Check sheet for the modelled part. Datum: model origin and axes. Units: mm. A direction names the side the tool comes from. Coordinates: 2 decimals unless noted, no trailing zeros. Write each loop counter-clockwise with the first axis right and the second up, starting at its lowest first coordinate (ties: lowest second). Pieces come first, ordered by that corner, then holes. Notation, with made-up numbers: (-12.75, -36.5) -> (-7.75, -36.5) arc R15 ccw to (-7.75, -27.5) -> close; hole circle Ø3 at (38.5, 28.25). An arc over 180 degrees is marked (long way). One line per item, written item: value. Start each with the question number.
1) Sectioned sample at C-C on z = -5. Enter the section's corners in (x, y).
2) Scan lines: line 1 along X through (y, z) = (14.5, -54.5); line 2 along X through (y, z) = (18, -39); line 3 along Y through (x, z) = (21.5, -45). Record each from-to range of solid material in increasing order. Write a range as [from, to].
3) Draft check along X on faces 1 (the flat face through (24, 35, -60.5)), 2 (the cylindrical face through (18.082, 14.392, -23.825)), 3 (the cylindrical face through (7.114, 14.392, -25.069)). Enter one of: +X half, -X half, draft (parallel to the pull), parting line (faces both ways), or undercut.
4) Sectioned sample at A-A on y = 34.5. Enter the section's corners in (x, z), plus the area to 3 significant figures.
5) Gauge pin test, flat ends, axial feed: P1, Ø4, axis at x = 45.5, z = -43, coming from the +Y side; P2, Ø1.5, axis at y = 51, z = -42, coming from the +X side; P3, Ø6.5, axis at x = 49.15, y = 18.55, coming from the +Z side. Record the tip position at first contact, or that the pin passes through.
6) Set-up check for faces 4 (the flat face through (14.65, 14.39, -25.02)), 5 (the flat face through (51, 5, -47)), 6 (the flat face through (16, 24.05, -52)): record each of +Z, -Z, +X, -X, +Y, -Y from which the full face is reachable in a straight line by a thin tool's end or side.
7) Sectioned sample at B-B on x = 11.5. Enter the section's corners in (y, z), plus the area to 3 significant figures.
```python
from build123d import *

# Parameters (mm, degrees)
BOSS_EXTRUDE1_DEPTH = 5
BOSS_EXTRUDE2_DEPTH = 5
BOSS_EXTRUDE3_DEPTH = 5
SKETCH6_R           = 2.5
CUT_EXTRUDE1_DEPTH  = 107.549284371
BOSS_EXTRUDE4_DEPTH = 19.05
SKETCH9_R           = 5.5
SKETCH9_R_2         = 2.5
BOSS_EXTRUDE5_DEPTH = 25.4


with BuildPart() as part:
    # Sketch1 → Boss-Extrude1 (new body)
    with BuildSketch(Plane(origin=(0, 0, 0), x_dir=(1, 0, 0), z_dir=(0, 1, 0))):
        Polygon((0, 0), (0, 60.5), (60.5, 60.5), (60.5, 47.75), (12.75, 0), align=None)
    extrude(amount=BOSS_EXTRUDE1_DEPTH)

    # Sketch4 → Boss-Extrude2 (add)
    with BuildSketch(Plane.ZY):
        Polygon((-60.5, 5), (-60.5, 68.5), (-19.4, 68.5), (0, 10.308629506), (0, 5), align=None)
    extrude(amount=-BOSS_EXTRUDE2_DEPTH)

    # Sketch5 → Boss-Extrude3 (add)
    with BuildSketch(Plane(origin=(0, 0, -60.5), x_dir=(-1, 0, 0), z_dir=(0, 0, -1))):
        Polygon((-5, 5), (-5, 68.5), (-41, 68.5), (-60.5, 10.004653177), (-60.5, 5), align=None)
    extrude(amount=-BOSS_EXTRUDE3_DEPTH)

    # Sketch6 → Cut-Extrude1 (cut, through all)
    with BuildSketch(Plane(origin=(0, 5, 0), x_dir=(1, 0, 0), z_dir=(0, 1, 0))):
        with Locations(Location((16.5, 15, 0), (0, 0, 270))):
            Circle(SKETCH6_R)
        with Locations(Location((45.5, 43, 0), (0, 0, 270))):
            Circle(SKETCH6_R)
    extrude(amount=-CUT_EXTRUDE1_DEPTH, mode=Mode.SUBTRACT)

    # Sketch7 → Boss-Extrude4 (add)
    with BuildSketch(Plane(origin=(0, 5, 0), x_dir=(1, 0, 0), z_dir=(0, 1, 0))):
        with BuildLine():
            Line((21.319247217, 19.543418849), (27.55028172, 14.80028172))
            Line((27.55028172, 14.80028172), (29.101515101, 16.351515101))
            ThreePointArc((29.101515101, 16.351515101), (24.666913521, 20.553458517), (19.305449591, 23.482062993))
            ThreePointArc((19.305449591, 23.482062993), (18.064972723, 23.830124106), (16.858784616, 24.282937146))
            Line((16.858784616, 24.282937146), (12.384629863, 25.774635894))
            ThreePointArc((12.384629863, 25.774635894), (11.23817984, 25.813438697), (10.255553875, 25.221577628))
            ThreePointArc((10.255553875, 25.221577628), (7.080749695, 25.107920962), (7.801379157, 28.201946269))
            ThreePointArc((7.801379157, 28.201946269), (8.483986824, 29.116932404), (8.624672831, 30.249787338))
            Line((8.624672831, 30.249787338), (7.827322243, 36.113739602))
            ThreePointArc((7.827322243, 36.113739602), (12.250646005, 48.939477405), (25.194853904, 53.00307497))
            Line((25.194853904, 53.00307497), (31.034265028, 52.042355532))
            ThreePointArc((31.034265028, 52.042355532), (32.170605503, 52.151365529), (33.104288638, 52.808167369))
            ThreePointArc((33.104288638, 52.808167369), (36.217223203, 53.44215303), (36.014993038, 50.271758357))
            ThreePointArc((36.014993038, 50.271758357), (35.395934706, 49.306035781), (35.402721719, 48.158949364))
            Line((35.402721719, 48.158949364), (36.768952902, 43.644900376))
            ThreePointArc((36.768952902, 43.644900376), (37.18792138, 42.426542952), (37.501221649, 41.17683405))
            ThreePointArc((37.501221649, 41.17683405), (40.195217667, 35.858711581), (44.131223781, 31.381223781))
            Line((44.131223781, 31.381223781), (45.737755925, 32.987755925))
            Line((45.737755925, 32.987755925), (41.382120343, 39.053882356))
            Line((41.382120343, 39.053882356), (41, 55.5))
            Line((41, 55.5), (32.491282289, 55.5))
            ThreePointArc((32.491282289, 55.5), (31.691168489, 54.800352321), (31.086863185, 53.925993089))
            ThreePointArc((31.086863185, 53.925993089), (29.049863177, 54.843826537), (26.91416103, 55.5))
            Line((26.91416103, 55.5), (5, 55.5))
            Line((5, 55.5), (5, 36.259130968))
            ThreePointArc((5, 36.259130968), (5.604814931, 33.17761818), (6.740301049, 30.249787338))
            ThreePointArc((6.740301049, 30.249787338), (5.763456299, 29.595667883), (5, 28.701669892))
            Line((5, 28.701669892), (5, 24.05684885))
            ThreePointArc((5, 24.05684885), (8.756409057, 22.076412717), (12.384629863, 24.282937146))
            Line((12.384629863, 24.282937146), (21.319247217, 19.543418849))
        make_face()
    extrude(amount=BOSS_EXTRUDE4_DEPTH)

    # Sketch9 → Boss-Extrude5 (add)
    with BuildSketch(Plane.XY.offset(-55.5)):
        with Locations(Location((49.152306284, 18.55, 0), (0, 0, 180))):
            Circle(SKETCH9_R)
        with Locations((49.152306284, 18.55)):
            Circle(SKETCH9_R_2, mode=Mode.SUBTRACT)
    extrude(amount=BOSS_EXTRUDE5_DEPTH)


solid = part.part
```
Answers:
1. outline: (0, 0) -> (17.75, 0) -> (17.75, 5) -> (5, 5) -> (5, 25.31) -> (0, 25.31) -> close
2. line 1: x = [0, 29.9], [31.45, 41.02], [45.43, 52.87]
2. line 2: x = [0, 7.71], [38.4, 41.42], [43.68, 46.71], [51.59, 54.62]
2. line 3: y = [0, 5]
3. face 1: draft
3. face 2: +X half
3. face 3: undercut
4. outline: (0, -60.5) -> (52.33, -60.5) -> (52.33, -55.5) -> (5, -55.5) -> (5, -8.06) -> (0, -8.06) -> close
4. area: 499 mm2
5. P1: stops at y = 23.8
5. P2: stops at x = 5
5. P3: stops at z = -30.1
6. face 4: +X, +Y
6. face 5: +X
6. face 6: +Z, +X, +Y
7. outline: (0, -60.5) -> (68.5, -60.5) -> (68.5, -55.5) -> (24.05, -55.5) -> (24.05, -48.15) -> (5, -48.15) -> (5, -25.86) -> (24.05, -25.86) -> (24.05, -23.18) -> (5, -23.18) -> (5, 0) -> (0, 0) -> close
7. area: 811 mm2
